```python
from build123d import *

# Parameters (mm, degrees)
SKETCH1_R                = 101.6
BOSS_EXTRUDE1_DEPTH      = 38.1
BOSS_EXTRUDE1_DEPTH_BACK = 38.1
SKETCH2_R                = 12.7
CUT_EXTRUDE1_DEPTH       = 76.2
FILLET1_R                = 25.4
SKETCH3_R                = 12.7
BOSS_EXTRUDE2_DEPTH      = 63.5
BOSS_EXTRUDE2_DEPTH_BACK = 63.5
SKETCH4_R                = 25.4
BOSS_EXTRUDE3_DEPTH      = 2.54
SKETCH5_R                = 25.4
BOSS_EXTRUDE4_DEPTH      = 2.54


with BuildPart() as part:
    # Sketch1 → Boss-Extrude1 (new body, two sides)
    with BuildSketch(Plane(origin=(0, 0, 0), x_dir=(1, 0, 0), z_dir=(0, 1, 0))) as boss_extrude1_sk:
        Circle(SKETCH1_R)
    extrude(amount=BOSS_EXTRUDE1_DEPTH)
    extrude(boss_extrude1_sk.sketch, amount=-BOSS_EXTRUDE1_DEPTH_BACK)

    # Sketch2 → Cut-Extrude1 (cut)
    with BuildSketch(Plane.XZ.offset(38.1)):
        Circle(SKETCH2_R)
    extrude(amount=-CUT_EXTRUDE1_DEPTH, mode=Mode.SUBTRACT)

    # Fillet1
    fillet1_edges = [part.edges().sort_by_distance(p)[0] for p in [
        (-101.6, 38.1, 0),
        (-101.6, -38.1, 0),
    ]]
    fillet(fillet1_edges, radius=FILLET1_R)

    # Sketch3 → Boss-Extrude2 (add, two sides)
    with BuildSketch(Plane(origin=(0, 0, 0), x_dir=(1, 0, 0), z_dir=(0, 1, 0))) as boss_extrude2_sk:
        Circle(SKETCH3_R)
    extrude(amount=BOSS_EXTRUDE2_DEPTH)
    extrude(boss_extrude2_sk.sketch, amount=-BOSS_EXTRUDE2_DEPTH_BACK)

    # Sketch4 → Boss-Extrude3 (add)
    with BuildSketch(Plane(origin=(0, 42.672, 0), x_dir=(1, 0, 0), z_dir=(0, 1, 0))):
        Circle(SKETCH4_R)
    boss_extrude3 = extrude(amount=BOSS_EXTRUDE3_DEPTH)

    # Sketch5 → Boss-Extrude4 (add)
    with BuildSketch(Plane(origin=(0, 41.402, 0), x_dir=(1, 0, 0), z_dir=(0, 1, 0))):
        Circle(SKETCH5_R)
    boss_extrude4 = extrude(amount=-BOSS_EXTRUDE4_DEPTH)

    # Mirror1: Boss-Extrude3, Boss-Extrude4 across plane
    add(boss_extrude3.mirror(Plane.ZX))
    add(boss_extrude4.mirror(Plane.ZX))


solid = part.part
```
For this review, take the finished solid that the model builds, in its own axes (mm). A direction names the side the tool comes from. Coordinates: 2 decimals unless noted, no trailing zeros. Write each loop counter-clockwise with the first axis right and the second up, starting at its lowest first coordinate (ties: lowest second). Pieces come first, ordered by that corner, then holes.
(1) The part is to be moulded in two halves that separate along Y. For faces 1 (the face through (5, 41.402, -12)), 2 (the face through (-22.025, 0.178, 99.184)), 3 (the face through (5, 45.212, -12)), say which applies: +Y half, -Y half, draft (parallel to the pull), parting line (faces both ways), or undercut.
(2) Add section A-A on y = 10. Give the boundary of the cut face in (x, z), then the cut area to 3 significant figures.
(3) Wall thickness on probe 1 along Y at (x, z) = (-18.5, 15); probe 2 along Y at (x, z) = (-36, 17); probe 3 along Y at (x, z) = (-57, -57.5): over which ranges is each line inside the solid? List them lowest first.
(4) For pin 1 Ø1.5 at (x, y) = (51, -2.5) entering from -Z; pin 2 Ø4 at (y, z) = (21.5, 4) entering from +X; pin 3 Ø3 at (x, z) = (74.5, 19) entering from +Y, all flat-tipped, find the tip position at first contact; note any pin that passes through.
(5) Tool access review of faces 4 (the face through (-2.75, -42.03, 12.4)), 5 (the face through (-5.506, 40.15, 24.796)), 6 (the face through (-5.506, -43.924, 24.796)): name each direction out of +Z, -Z, +X, -X, +Y, -Y from which nothing blocks a thin tool from reaching the whole face with its end or side.
(6) Add section B-B on y = 50. Give the boundary of the cut face in (x, z), then the cut area to 3 significant figures.
Answer sheet:
1. face 1: undercut
1. face 2: draft
1. face 3: +Y half
2. outline: circle Ø203.2 at (0, 0)
2. area: 32,400 mm2
3. probe 1: y = -45.21 to -42.67, -41.4 to -38.86, -38.1 to 38.1, 38.86 to 41.4, 42.67 to 45.21
3. probe 2: y = -38.1 to 38.1
3. probe 3: y = -37.65 to 37.65
4. pin 1: stops at z = -88.3
4. pin 2: stops at x = 100.6
4. pin 3: stops at y = 38.1
5. face 4: none
5. face 5: +Y
5. face 6: -Y
6. outline: circle Ø25.4 at (0, 0)
6. area: 507 mm2
